from build123d import *

# Parameters (mm, degrees)
SKETCH1_R           = 15.5
BOSS_EXTRUDE1_DEPTH = 30
SKETCH2_R           = 14
CUT_EXTRUDE1_DEPTH  = 27
SKETCH3_R           = 1
CUT_EXTRUDE2_DEPTH  = 10
SKETCH4_R           = 3.75
BOSS_EXTRUDE2_DEPTH = 27


with BuildPart() as part:
    # Sketch1 → Boss-Extrude1 (new body)
    with BuildSketch(Plane(origin=(0, 0, 0), x_dir=(1, 0, 0), z_dir=(0, 1, 0))):
        with Locations(Location((0, 0, 0), (0, 0, 270))):
            Circle(SKETCH1_R)
    extrude(amount=BOSS_EXTRUDE1_DEPTH)

    # Sketch2 → Cut-Extrude1 (cut)
    with BuildSketch(Plane(origin=(0, 30, 0), x_dir=(1, 0, 0), z_dir=(0, 1, 0))):
        with Locations(Location((0, 0, 0), (0, 0, 270))):
            Circle(SKETCH2_R)
    extrude(amount=-CUT_EXTRUDE1_DEPTH, mode=Mode.SUBTRACT)

    # Sketch3 → Cut-Extrude2 (cut)
    with BuildSketch(Plane.XZ):
        with Locations(Location((-9, 0, 0), (0, 0, 270))):
            Circle(SKETCH3_R)
        with Locations(Location((-12.5, 0, 0), (0, 0, 270))):
            Circle(SKETCH3_R)
    extrude(amount=-CUT_EXTRUDE2_DEPTH, mode=Mode.SUBTRACT)

    # Sketch4 → Boss-Extrude2 (add)
    with BuildSketch(Plane(origin=(0, 3, 0), x_dir=(1, 0, 0), z_dir=(0, 1, 0))):
        with Locations(Location((0, 0, 0), (0, 0, 270))):
            Circle(SKETCH4_R)
    extrude(amount=BOSS_EXTRUDE2_DEPTH)


solid = part.part
Check sheet for the modelled part. Datum: model origin and axes. Units: mm. A direction names the side the tool comes from. Round coordinates to 2 decimals unless told otherwise and drop trailing zeros. Loops run counter-clockwise (first coordinate to the right, second up) from the corner with the lowest first, then second, coordinate; pieces in that order, holes last. Notation, with made-up numbers: (15.5, -9) - (20.5, -9) arc R32 cw to (20.5, 30) - close; hole circle Ø1 at (69.25, 39.25). An arc over 180 degrees is marked (long way). Answer as CSV lines item,"result". Start each with the question number.
Item 1: Section check C-C (x = 0). Record the boundary of the cut face in (y, z).
Item 2: Scan lines: line 1 (X direction, y = 0.7, z = 0); line 2 (Z direction, x = 1, y = 8.25); line 3 (Z direction, x = -3, y = 3.75). Record each from-to range of solid material in increasing order. Write a range as [from, to].
Item 3: Section check B-B (x = -9). Record the boundary of the cut face in (y, z).
Item 4: Set-up check for faces 1 (the cylindrical face through (-13.1, 1.5, 0.8)), 2 (the flat face through (-3, 3, 3)): record each of +Z, -Z, +X, -X, +Y, -Y from which the full face is reachable in a straight line by a thin tool's end or side.
Item 5: Section check D-D (z = 6). Record the boundary of the cut face in (x, y).
Item 6: Release check for a two-part mould opening along Z. For faces 3 (the cylindrical face through (-8, 1, 0)), 4 (the flat face through (0, 0, 0)), 5 (the cylindrical face through (15.368, 14.79, -2.018)) record: +Z half, -Z half, draft (parallel to the pull), parting line (faces both ways), or undercut.
Item 7: Section check A-A (y = 16.25). Record the boundary of the cut face in (x, z).
Item 8: Depth check by flat-ended pin: P1, Ø3, axis at y = 27, z = 9.5, coming from the +X side; P2, Ø2, axis at x = -4.5, y = 7.5, coming from the +Z side; P3, Ø8, axis at x = 11.5, y = 7.5, coming from the +Z side. Enter the tip coordinate at first touch or a pass-through.
Report:
1,outline,"(0, -15.5) - (30, -15.5) - (30, -14) - (3, -14) - (3, -3.75) - (30, -3.75) - (30, 3.75) - (3, 3.75) - (3, 14) - (30, 14) - (30, 15.5) - (0, 15.5) - close"
2,line 1,"x = [-15.5, -13.5], [-11.5, -10], [-8, 15.5]"
2,line 2,"z = [-15.47, -13.96], [-3.61, 3.61], [13.96, 15.47]"
2,line 3,"z = [-15.21, -13.67], [-2.25, 2.25], [13.67, 15.21]"
3,outline,"(0, -12.62) - (30, -12.62) - (30, -10.72) - (3, -10.72) - (3, -1) - (0, -1) - close; (0, 1) - (3, 1) - (3, 10.72) - (30, 10.72) - (30, 12.62) - (0, 12.62) - close"
4,face 1,"+Y, -Y"
4,face 2,"+Y"
5,outline,"(-14.29, 0) - (14.29, 0) - (14.29, 30) - (12.65, 30) - (12.65, 3) - (-12.65, 3) - (-12.65, 30) - (-14.29, 30) - close"
6,face 3,"undercut"
6,face 4,"draft"
6,face 5,"parting line"
7,outline,"circle Ø31 at (0, 0); circle Ø7.5 at (0, 0); hole circle Ø28 at (0, 0)"
8,P1,"stops at x = 13.28"
8,P2,"stops at z = 15.1"
8,P3,"stops at z = 13.56"
